Can you work these out from the drawing? Everything is in mm from the part's minimum corner. A direction names the side the tool comes from. Give positions to 0.01 mm unless a question says otherwise; leave off trailing zeros. One line per item, written item: value.
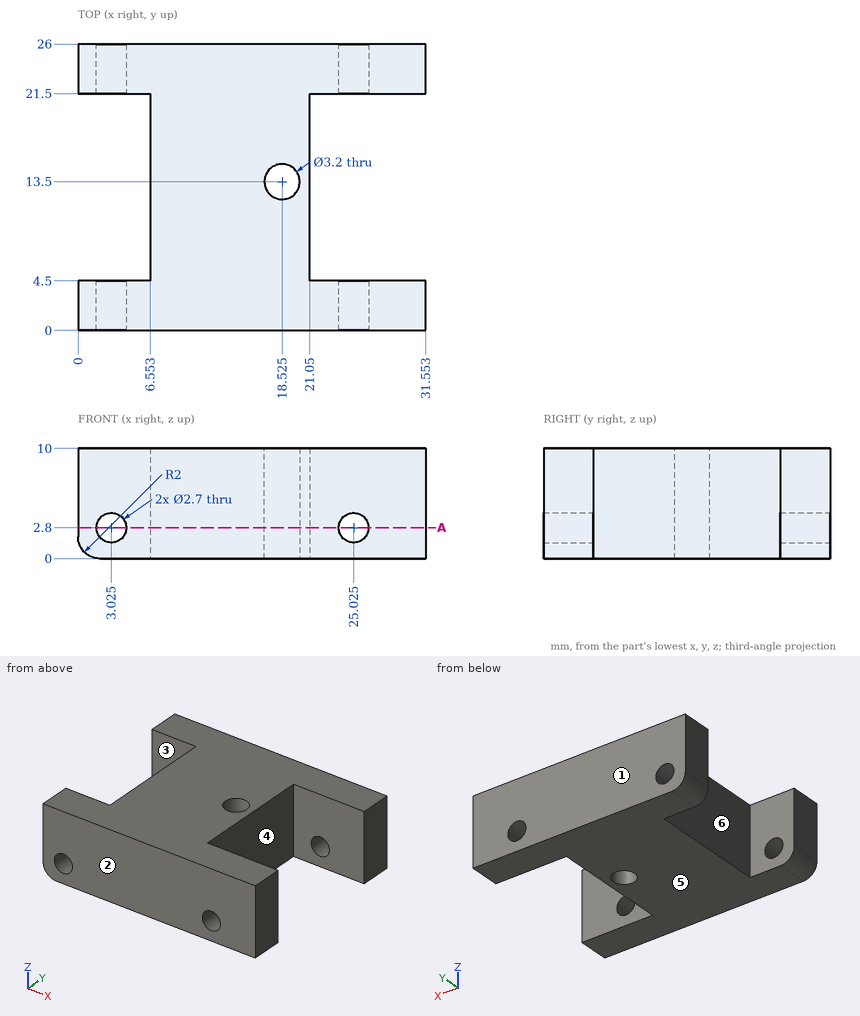
1) We'd pull the mould along Y, two halves only. Please class the marked faces 1, 2 and 3: pulls with the +Y half, pulls with the -Y half, needs draft (parallel to the pull), parting line crosses it, or undercut.
Outcome:
face 1: pulls with the +Y half
face 2: pulls with the -Y half
face 3: undercut
2) On a 3-axis mill with a long thin cutter (end or side, diameter ignored), from which of +Z, -Z, +X, -X, +Y, -Y can I reach the whole of each face in a straight line? I mean the marked faces 4, 5 and 6. Say none if no direction works.
Outcome:
face 4: +Z, -Z, +X
face 5: -Z, +X, -X, +Y, -Y
face 6: +Z, -Z, -X
3) Please list where these lines run through material, in increasing order: L1, parallel to X at y = 1.15, z = 2.8 (1 decimal); L2, parallel to Y at x = 5, z = 6.25; L3, parallel to Z at x = 24.5, y = 2 (1 decimal). Write a range as from..to.
Outcome:
L1: x = 0..1.7, 4.4..23.7, 26.4..31.6
L2: y = 0..4.5, 21.5..26
L3: z = 0..1.6, 4..10
4) If we section it at A-A, the plane z = 2.8: Give the number of separate pieces and of enclosed holes in the cut face, then the cut area to 3 significant figures.
Outcome:
separate pieces: 5
enclosed holes: 1
area: 474 mm^2
5) I'm going to push flat-ended pins straight in: pin 1 (2 mm diameter, centred on x = 3.025, z = 2.8, fed in from -Y); pin 2 (5 mm diameter, centred on y = 18.5, z = 2.5, fed in from -X); pin 3 (1 mm diameter, centred on y = 4.5, z = 3.5, fed in from -X). Where does each tip first touch, or does it pass through?
Outcome:
pin 1: passes through
pin 2: stops at x = 6.55
pin 3: stops at x = 0
